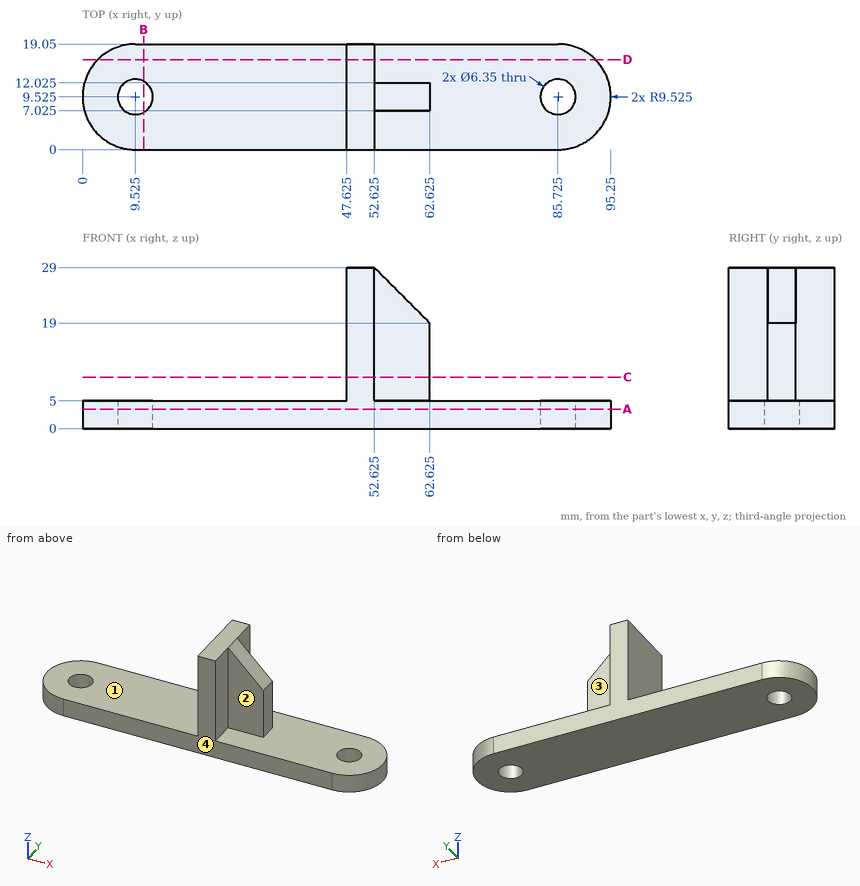
Source: three-view drawing plus pictorial views. Frame: mm from the lowest corner of the part. A direction names the side the tool comes from. Give positions to 0.01 mm unless a question says otherwise; leave off trailing zeros. Order: outer loops, then holes, each group sorted by start corner. A loop starts at its lowest first (then second) coordinate and runs counter-clockwise, first axis right, second up.
1. Reachability of the marked faces 1, 2, 3 and 4 from +Z, -Z, +X, -X, +Y, -Y: full face, straight path, thin tool, end or side. Return the list, or none.
Derived:
face 1: +Z, -X, +Y, -Y
face 2: +Z, +X, -Y
face 3: +Z, +X, +Y
face 4: +Z, -Z, +X, -X, -Y
2. Section D-D on y = 16.25. Return the cut outline in (x, z) (3 decimals), and give its area (3 significant figures).
Derived:
outline: (2.78, 0) - (92.47, 0) - (92.47, 5) - (52.625, 5) - (52.625, 29) - (47.625, 29) - (47.625, 5) - (2.78, 5) - close
area: 568 mm2
3. Section A-A on z = 3.5. Return the cut outline in (x, y) (3 decimals).
Derived:
outline: (9.525, 0) - (85.725, 0) arc R9.525 ccw to (85.725, 19.05) - (9.525, 19.05) arc R9.525 ccw to start; hole circle Ø6.35 at (9.525, 9.525); hole circle Ø6.35 at (85.725, 9.525)
4. Material intervals for L1, parallel to X at y = 8.5, z = 4.5; L2, parallel to Z at x = 13.5, y = 6.25; L3, parallel to X at y = 14, z = 18 (3 decimals), sorted ascending.
Derived:
L1: x = 0.06 to 6.52, 12.53 to 82.72, 88.73 to 95.19
L2: z = 0 to 5
L3: x = 47.625 to 52.625
5. Section B-B on x = 11. Return the cut outline in (y, z).
Derived:
outline: (0, 0) - (6.71, 0) - (6.71, 5) - (0, 5) - close; (12.34, 0) - (19.05, 0) - (19.05, 5) - (12.34, 5) - close
6. Section C-C on z = 9.25. Return the cut outline in (x, y) (3 decimals), and give its area (3 significant figures).
Derived:
outline: (47.625, 0) - (52.625, 0) - (52.625, 7.025) - (62.625, 7.025) - (62.625, 12.025) - (52.625, 12.025) - (52.625, 19.05) - (47.625, 19.05) - close
area: 145 mm2
7. Pin query (flat end, axial travel): pin 1 (5.5 mm diameter, centred on x = 9.525, y = 9.525, fed in from +Z); pin 2 (8 mm diameter, centred on x = 73.5, y = 4, fed in from +Z); pin 3 (11 mm diameter, centred on x = 58.5, z = 18, fed in from +Y) (3 decimals); pin 4 (10 mm diameter, centred on x = 27.5, y = 4.5, fed in from -Z). Return the tip coordinate at first contact, or that it passes through.
Derived:
pin 1: passes through
pin 2: stops at z = 5
pin 3: stops at y = 12.025
pin 4: stops at z = 0
